For this review, use the dimensioned drawing (mm, ordinates from the lowest corner) and the shaded views. Coordinates: 2 decimals unless noted, no trailing zeros. Write each loop counter-clockwise with the first axis right and the second up, starting at its lowest first coordinate (ties: lowest second). Pieces come first, ordered by that corner, then holes. Notation, with made-up numbers: (-29.75, -22.5) - (-8.75, -22.5) arc R30 cw to (-8.75, 0.5) - close; hole circle Ø3 at (77.5, 48). An arc over 180 degrees is marked (long way). Use one line per item in the form item = value. Start each with the question number.
1) Insertion check: P1, Ø8, axis at x = 96.5, y = 12.5, coming from the -Z side; P2, Ø1.5, axis at x = 21, z = 54, coming from the +Y side. Each pin has a flat end and moves straight along its axis. Give the tip position at first contact, or say it passes through.
2) We need section B-B (z = 76). Give the boundary of the cut face in (x, y), plus the area to 4 significant figures.
3) We need section A-A (y = 5.75). Give the boundary of the cut face in (x, z).
4) We need section D-D (y = 21). Give the boundary of the cut face in (x, z), plus the area to 3 significant figures.
5) We need section C-C (x = 83). Give the boundary of the cut face in (y, z), plus the area to 3 significant figures.
6) For L1, parallel to Z at x = 46.5, y = 22; L2, parallel to X at y = 19.25, z = 28; L3, parallel to X at y = 21, z = 5.5, list the stretches that pass through material, from the lowest coordinate up. Write a range as from..to.
7) Mouldability with a two-part tool opening along X and no side actions: class the marked faces 1, 2, 3 and 4 as pulls with the +X half, pulls with the -X half, needs draft (parallel to the pull), parting line crosses it, or undercut.
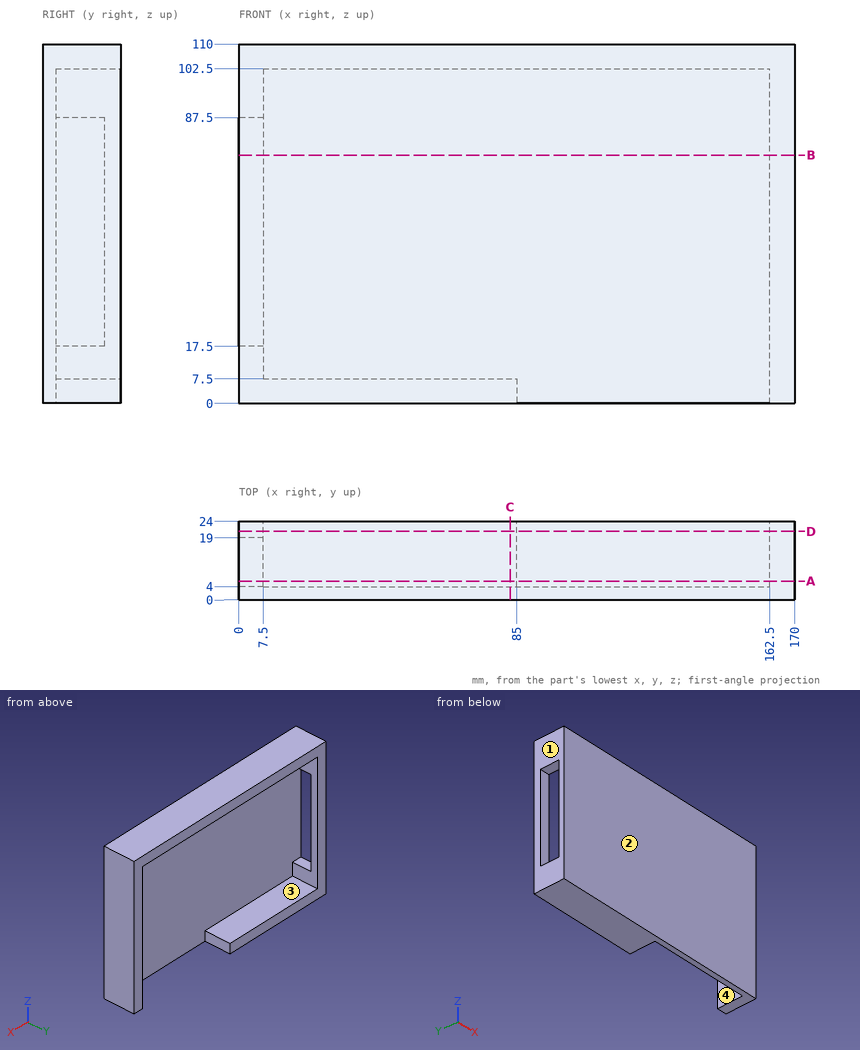
Determined:
q1.P1 = 102.5
q1.P2 = 4
q2.outline = (0, 0) - (170, 0) - (170, 24) - (162.5, 24) - (162.5, 4) - (0, 4) - close; (0, 19) - (7.5, 19) - (7.5, 24) - (0, 24) - close
q2.area = 867.5 mm²
q3.outline = (0, 0) - (85, 0) - (85, 7.5) - (7.5, 7.5) - (7.5, 17.5) - (0, 17.5) - close; (0, 87.5) - (7.5, 87.5) - (7.5, 102.5) - (162.5, 102.5) - (162.5, 0) - (170, 0) - (170, 110) - (0, 110) - close
q4.outline = (0, 0) - (85, 0) - (85, 7.5) - (7.5, 7.5) - (7.5, 102.5) - (162.5, 102.5) - (162.5, 0) - (170, 0) - (170, 110) - (0, 110) - close
q4.area = 3,390 mm²
q5.outline = (0, 0) - (24, 0) - (24, 7.5) - (4, 7.5) - (4, 102.5) - (24, 102.5) - (24, 110) - (0, 110) - close
q5.area = 740 mm²
q6.L1 = 0..7.5, 102.5..110
q6.L2 = 0..7.5, 162.5..170
q6.L3 = 0..85, 162.5..170
q7.face_1 = pulls with the -X half
q7.face_2 = needs draft
q7.face_3 = undercut
q7.face_4 = undercut
